Geometry: final body of the model. Coordinates: model frame, mm. Face numbers are marked on the shaded views. A direction names the side the tool comes from. Round coordinates to 2 decimals unless told otherwise and drop trailing zeros. Loops run counter-clockwise (first coordinate to the right, second up) from the corner with the lowest first, then second, coordinate; pieces in that order, holes last. Notation, with made-up numbers: (34, -19.5) - (40, -19.5) arc R37 cw to (40, 17.5) - close; hole circle Ø1 at (0.5, -9.5). An arc over 180 degrees is marked (long way). Answer as a JSON object with one key per item and string values. Group by question number.
Item 1: Section B-B (z = 34.5). Return the cut outline in (x, y), plus the area to 3 significant figures.
Item 2: Section A-A (x = -21.5). Return the cut outline in (y, z).
Item 3: First-contact query: pin 1 (4 mm diameter, centred on x = -11.5, y = -3, fed in from -Z); pin 2 (4 mm diameter, centred on y = -6.5, z = 29, fed in from +X); pin 3 (1 mm diameter, centred on y = -6, z = 18.5, fed in from -X). Flat tips, straight axial feed; report the tip coordinate or a pass-through.
Item 4: Line query: line 1 (X direction, y = -2.25, z = -16); line 2 (X direction, y = -1.5, z = 9); line 3 (Z direction, x = 26.5, y = -4.25). Output: solid intervals per line, ascending.
Item 5: Section C-C (x = 0). Return the cut outline in (y, z).
Item 6: Reachability of the marked faces 1 and 2 from +Z, -Z, +X, -X, +Y, -Y: full face, straight path, thin tool, end or side. Return the list, or none.
Item 7: Section D-D (y = -5.5). Count the separate pieces of the cut face and the enclosed holes in it, plus the area to 3 significant figures.
Item 8: Draft query along Z for the marked faces 3, 4 and 5. Return one class per face: released by +Z, released by -Z, zero draft, split by the parting line, or undercut.
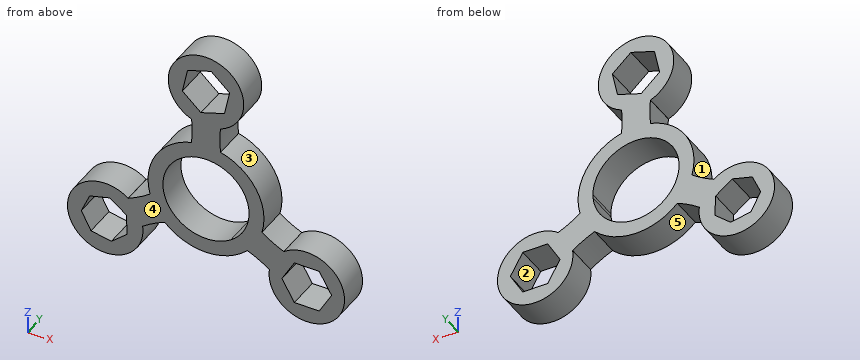
```python
from build123d import *

# Parameters (mm, degrees)
F1_DEPTH = 8


with BuildPart() as f1:
    # F0 (on Front) → F1 (new body)
    with BuildSketch(Plane.XZ):
        with BuildLine():
            ThreePointArc((3.672208, 20.620274), (0, 38.993878), (-3.672208, 20.620274))
            Line((-3.672208, 20.620274), (-3.672208, 20.747529))
            ThreePointArc((-3.672208, 20.747529), (-3.664311, 20.680667), (-3.656581, 20.613784))
            ThreePointArc((-3.656581, 20.613784), (-3.482802, 17.406357), (-3.692215, 14.201059))
            ThreePointArc((-3.692215, 14.201059), (-12.707356, 7.336596), (-14.144586, -3.902978))
            ThreePointArc((-14.144586, -3.902978), (-16.815748, -5.686984), (-19.680351, -7.1402))
            ThreePointArc((-19.680351, -7.1402), (-19.742138, -7.166947), (-19.803991, -7.19354))
            Line((-19.803991, -7.19354), (-19.693785, -7.129912))
            ThreePointArc((-19.693785, -7.129912), (-33.769689, -19.496939), (-16.021578, -13.490362))
            Line((-16.021578, -13.490362), (-16.131784, -13.55399))
            ThreePointArc((-16.131784, -13.55399), (-16.077827, -13.51372), (-16.02377, -13.473584))
            ThreePointArc((-16.02377, -13.473584), (-13.332947, -11.719373), (-10.452371, -10.298081))
            ThreePointArc((-10.452371, -10.298081), (0, -14.673191), (10.452371, -10.298081))
            ThreePointArc((10.452371, -10.298081), (13.332947, -11.719373), (16.02377, -13.473584))
            ThreePointArc((16.02377, -13.473584), (16.077827, -13.51372), (16.131784, -13.55399))
            Line((16.131784, -13.55399), (16.021578, -13.490362))
            ThreePointArc((16.021578, -13.490362), (33.769689, -19.496939), (19.693785, -7.129912))
            Line((19.693785, -7.129912), (19.803991, -7.19354))
            ThreePointArc((19.803991, -7.19354), (19.742138, -7.166947), (19.680351, -7.1402))
            ThreePointArc((19.680351, -7.1402), (16.815748, -5.686984), (14.144586, -3.902978))
            ThreePointArc((14.144586, -3.902978), (12.707356, 7.336596), (3.692215, 14.201059))
            ThreePointArc((3.692215, 14.201059), (3.482802, 17.406357), (3.656581, 20.613784))
            ThreePointArc((3.656581, 20.613784), (3.664311, 20.680667), (3.672208, 20.747529))
            Line((3.672208, 20.747529), (3.672208, 20.620274))
        make_face()
        Polygon((-23.943451, -20.566496), (-29.098889, -19.578989), (-31.541188, -14.932604), (-29.431247, -10.126165), (-24.357895, -8.779017), (-20.141468, -11.90559), (-19.957023, -17.151512), align=None, mode=Mode.SUBTRACT)
        Polygon((31.788998, -14.720053), (28.642439, -20.170053), (22.349321, -20.170053), (19.202762, -14.720053), (22.349321, -9.270053), (28.642439, -9.270053), align=None, mode=Mode.SUBTRACT)
        with BuildLine():
            ThreePointArc((10.9, 0), (10.889444, -0.479582), (10.857798, -0.958236))
            ThreePointArc((10.857798, -0.958236), (9.439677, -5.45), (6.258756, -8.924011))
            ThreePointArc((6.258756, -8.924011), (-9.670327, 5.029392), (10.9, 0))
        make_face(mode=Mode.SUBTRACT)
        Polygon((4.68163, 25.234673), (-1.301197, 23.282979), (-5.982827, 27.488413), (-4.68163, 33.64554), (1.301197, 35.597234), (5.982827, 31.391801), align=None, mode=Mode.SUBTRACT)
        with BuildLine():
            Line((-3.672208, 20.747529), (-3.672208, 20.620274))
            ThreePointArc((-3.672208, 20.620274), (-3.664396, 20.617026), (-3.656581, 20.613784))
            ThreePointArc((-3.656581, 20.613784), (-3.664311, 20.680667), (-3.672208, 20.747529))
        make_face()
        with BuildLine():
            ThreePointArc((3.656581, 20.613784), (3.664396, 20.617026), (3.672208, 20.620274))
            Line((3.672208, 20.620274), (3.672208, 20.747529))
            ThreePointArc((3.672208, 20.747529), (3.664311, 20.680667), (3.656581, 20.613784))
        make_face()
        with BuildLine():
            ThreePointArc((-19.803991, -7.19354), (-19.742138, -7.166947), (-19.680351, -7.1402))
            ThreePointArc((-19.680351, -7.1402), (-19.687066, -7.135053), (-19.693785, -7.129912))
            Line((-19.693785, -7.129912), (-19.803991, -7.19354))
        make_face()
        with BuildLine():
            ThreePointArc((19.693785, -7.129912), (19.687066, -7.135053), (19.680351, -7.1402))
            ThreePointArc((19.680351, -7.1402), (19.742138, -7.166947), (19.803991, -7.19354))
            Line((19.803991, -7.19354), (19.693785, -7.129912))
        make_face()
        with BuildLine():
            Line((-16.131784, -13.55399), (-16.021578, -13.490362))
            ThreePointArc((-16.021578, -13.490362), (-16.02267, -13.481973), (-16.02377, -13.473584))
            ThreePointArc((-16.02377, -13.473584), (-16.077827, -13.51372), (-16.131784, -13.55399))
        make_face()
        with BuildLine():
            ThreePointArc((16.02377, -13.473584), (16.02267, -13.481973), (16.021578, -13.490362))
            Line((16.021578, -13.490362), (16.131784, -13.55399))
            ThreePointArc((16.131784, -13.55399), (16.077827, -13.51372), (16.02377, -13.473584))
        make_face()
    extrude(amount=F1_DEPTH)


solid = f1.part
```
Values:
{
 "1": {"outline": "(-8.1, -8) - (-2.06, -8) - (-2.06, 0) - (-8.1, 0) - close; (2.52, -8) - (8.1, -8) - (8.1, 0) - (2.52, 0) - close", "area": "93.0 mm^2"},
 "2": {"outline": "(-8, -23.4) - (0, -23.4) - (0, -18.47) - (-8, -18.47) - close; (-8, -10.9) - (0, -10.9) - (0, -6.04) - (-8, -6.04) - close"},
 "3": {"pin 1": "stops at z = -11.82", "pin 2": "stops at x = 9.55", "pin 3": "stops at x = -3.52"},
 "4": {"line 1": "x = -34.96 to -30.98, -20 to -16.03, 16.03 to 19.94, 31.05 to 34.96", "line 2": "x = -11.59 to -6.15, 6.15 to 11.59", "line 3": "z = -24.22 to -20.17, -9.27 to -5.22"},
 "5": {"outline": "(-8, -14.67) - (0, -14.67) - (0, -10.9) - (-8, -10.9) - close; (-8, 10.9) - (0, 10.9) - (0, 23.71) - (-8, 23.71) - close; (-8, 35.17) - (0, 35.17) - (0, 38.99) - (-8, 38.99) - close"},
 "6": {"face 1": "-X, +Y, -Y", "face 2": "+Y, -Y"},
 "7": {"separate pieces": "1", "enclosed holes": "4", "area": "976 mm^2"},
 "8": {"face 3": "undercut", "face 4": "zero draft", "face 5": "released by -Z"}
}
